Can you work these out from the model? Positions are in its coordinate system, mm. Give positions to 0.01 mm unless a question says otherwise; leave off trailing zeros. Order: outer loops, then holes, each group sorted by start corner. A loop starts at its lowest first (then second) coordinate and runs counter-clockwise, first axis right, second up. Notation, with made-up numbers: M 83,89.5 L 140,89.5 A22 ccw 140,107.5 Z; hole C -29.75,-4.75 d8. An arc over 180 degrees is marked long. One line per question, with ' | ' between items. Start each with the question number.
1) If we section it at D-D, the plane x = 46.5: Please give me the cut outline in (y, z), plus the area to 3 significant figures.
2) If we section it at A-A, the plane x = 34: Please give me the cut outline in (y, z).
3) If we section it at C-C, the plane y = 0.75: State how many separate pieces and enclosed holes the cut face has, plus the area to 3 significant figures.
4) If we section it at B-B, the plane x = 17: Please give me the cut outline in (y, z), plus the area to 3 significant figures.
5) Please list where these lines run through material, in increasing order: line 1 along Z through (x, y) = (23, 0.25); line 2 along Z through (x, y) = (26.5, 2.05); line 3 along X through (y, z) = (1.9, 38.5). Write a range as [from, to].
6) I'm going to push flat-ended pins straight in: pin 1 Ø1.5 at (x, y) = (30, 2) entering from -Z; pin 2 Ø1 at (y, z) = (2, -22) entering from +X; pin 3 Ø1.5 at (x, y) = (32.5, 1) entering from +Z. Where does each tip first touch, or does it pass through?
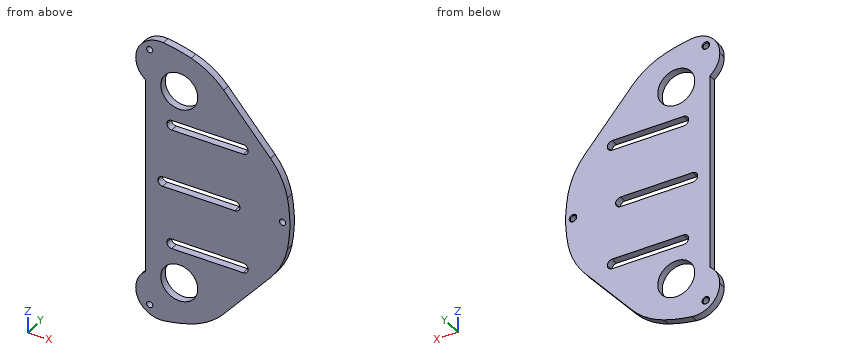
```python
from build123d import *

# Parameters (mm, degrees)
EXTRUDE_1_DEPTH              = 3
FILLET_1_R                   = 10
SKETCH_2_W                   = 33
SKETCH_2_H                   = 4
SKETCH_2_W_2                 = 33.308993126
CUT_EXTRUDE_1_DEPTH          = 83.523019213
SKETCH_3_W                   = 8
SKETCH_3_H                   = 80
CUT_EXTRUDE_2_DEPTH          = 83.523019213
FILLET_2_R                   = 10
FILLET_3_R                   = 2
CUT_EXTRUDE_3_DEPTH          = 83.523019213
FILLET_4_R                   = 30
SKETCH_5_R                   = 7.5
CUT_EXTRUDE_4_DEPTH          = 83.523019213
HOLE_WIZARD_M3_1_D           = 2.5
HOLE_WIZARD_M3_1_DEPTH       = 3
HOLE_WIZARD_M3_1_CSINK_D     = 3.05
HOLE_WIZARD_M3_1_CSINK_ANGLE = 90
HOLE_WIZARD_M3_1_TIP         = 0.751075774


# Some blends are built 0.0001 mm under size
with BuildPart() as part:
    # 草图1 → 凸台-拉伸1 (new body)
    with BuildSketch(Plane(origin=(0, 0, 0), x_dir=(1, 0, 0), z_dir=(0, 1, 0))):
        with BuildLine():
            Line((-4, 58.36308765), (-4, -58.36308765))
            ThreePointArc((-4, -58.36308765), (58.5, 0), (-4, 58.36308765))
        make_face()
    extrude(amount=EXTRUDE_1_DEPTH)

    # 圆角1
    fillet_1_edges = [part.edges().sort_by_distance(p)[0] for p in [
        (-4, 1.5, 58.36308765),
        (-4, 1.5, -58.36308765),
    ]]
    fillet(fillet_1_edges, radius=FILLET_1_R)

    # 草图2 → 切除-拉伸1 (cut, through all)
    with BuildSketch(Plane.XZ):
        with Locations((25.103538951, 24.75)):
            Rectangle(SKETCH_2_W, SKETCH_2_H)
        with Locations((25.103538951, -24.75)):
            Rectangle(SKETCH_2_W, SKETCH_2_H)
        with Locations((21.59426648, 0)):
            Rectangle(SKETCH_2_W_2, SKETCH_2_H)
    extrude(amount=-CUT_EXTRUDE_1_DEPTH, mode=Mode.SUBTRACT)

    # 草图3 → 切除-拉伸2 (cut, through all)
    with BuildSketch(Plane.XZ):
        with Locations((-4, 0)):
            Rectangle(SKETCH_3_W, SKETCH_3_H)
    extrude(amount=-CUT_EXTRUDE_2_DEPTH, mode=Mode.SUBTRACT)

    # 圆角2
    # the kernel refuses this fillet: 10 mm, written as the material it takes off along each edge
    with BuildSketch(Plane(origin=(-4, 23, 40), x_dir=(0, 0, 1), z_dir=(0, -1, 0)), Plane(origin=(-4, -20, -40), x_dir=(0, 0, -1), z_dir=(0, 1, 0))) as fillet_2_piece_1:
        with BuildLine():
            CenterArc((8, -10), FILLET_2_R, 90, 53.130102354)
            Line((0, -4), (-0.16, -3.88))
            ThreePointArc((-0.16, -3.88), (-0.2, -2), (-0.2, 0))
            Line((-0.2, 0), (0, 0.2))
            Line((0, 0.2), (8, 0.2))
            Line((8, 0.2), (8, 0))
        make_face()
    extrude(amount=43, mode=Mode.SUBTRACT)

    # 圆角3
    fillet_3_edges = [part.edges().sort_by_distance(p)[0] for p in [
        (8.603538951, 1.5, -26.75),
        (8.603538951, 1.5, -22.75),
        (41.603538951, 1.5, -26.75),
        (41.603538951, 1.5, -22.75),
        (4.939769917, 1.5, 2),
        (38.248763043, 1.5, 2),
        (38.248763043, 1.5, -2),
        (4.939769917, 1.5, -2),
        (41.603538951, 1.5, 22.75),
        (41.603538951, 1.5, 26.75),
        (8.603538951, 1.5, 22.75),
        (8.603538951, 1.5, 26.75),
    ]]
    fillet(fillet_3_edges, radius=FILLET_3_R - 0.0001)  # a hair under: the kernel refuses the full size

    # 草图4 → 切除-拉伸3 (cut, through all)
    with BuildSketch(Plane(origin=(0, 3, 0), x_dir=(1, 0, 0), z_dir=(0, 1, 0))):
        with BuildLine():
            Line((55.026651821, -19.857431591), (27.299740921, -51.73948343))
            ThreePointArc((27.299740921, -51.73948343), (44.142100571, -38.389125506), (55.026651821, -19.857431591))
        make_face()
        with BuildLine():
            Line((55.026651821, 19.857431591), (27.299740921, 51.73948343))
            ThreePointArc((27.299740921, 51.73948343), (44.142100571, 38.389125506), (55.026651821, 19.857431591))
        make_face()
    extrude(amount=-CUT_EXTRUDE_3_DEPTH, mode=Mode.SUBTRACT)

    # 圆角4
    fillet_4_edges = [part.edges().sort_by_distance(p)[0] for p in [
        (55.026651821, 1.5, 19.857431591),
        (27.299740921, 1.5, 51.73948343),
        (27.299740921, 1.5, -51.73948343),
        (55.026651821, 1.5, -19.857431591),
    ]]
    fillet(fillet_4_edges, radius=FILLET_4_R)

    # 草图5 → 切除-拉伸4 (cut, through all)
    with BuildSketch(Plane(origin=(0, 3, 0), x_dir=(1, 0, 0), z_dir=(0, 1, 0))):
        with Locations(Location((13.650269614, 40, 0), (0, 0, 270))):
            Circle(SKETCH_5_R)
        with Locations(Location((13.650269614, -40, 0), (0, 0, 270))):
            Circle(SKETCH_5_R)
    extrude(amount=-CUT_EXTRUDE_4_DEPTH, mode=Mode.SUBTRACT)

    # M3 螺纹孔1
    with Locations(Plane(origin=(0, 3, 0), x_dir=(1, 0, 0), z_dir=(0, 1, 0))):
        with Locations((1.668639438, 53.213363577), (1.668639438, -53.213363577), (0.79229906, -68.463573452), (55.526064592, 0.086594156)):
            CounterSinkHole(HOLE_WIZARD_M3_1_D / 2, HOLE_WIZARD_M3_1_CSINK_D / 2, depth=HOLE_WIZARD_M3_1_DEPTH, counter_sink_angle=HOLE_WIZARD_M3_1_CSINK_ANGLE)
            with Locations((0, 0, -(HOLE_WIZARD_M3_1_DEPTH + HOLE_WIZARD_M3_1_TIP / 2))):  # 118° drill point
                Cone(0, HOLE_WIZARD_M3_1_D / 2, HOLE_WIZARD_M3_1_TIP, mode=Mode.SUBTRACT)


solid = part.part
```
Results found:
1) outline: M 0,-29.66 L 3,-29.66 L 3,29.66 L 0,29.66 Z | area: 178 mm²
2) outline: M 0,-44.04 L 3,-44.04 L 3,-26.75 L 0,-26.75 Z; M 0,-22.75 L 3,-22.75 L 3,-2 L 0,-2 Z; M 0,2 L 3,2 L 3,22.75 L 0,22.75 Z; M 0,26.75 L 3,26.75 L 3,44.04 L 0,44.04 Z
3) separate pieces: 1 | enclosed holes: 8 | area: 4,460 mm²
4) outline: M 0,-55.98 L 3,-55.98 L 3,-46.71 L 0,-46.71 Z; M 0,-33.29 L 3,-33.29 L 3,-26.75 L 0,-26.75 Z; M 0,-22.75 L 3,-22.75 L 3,-2 L 0,-2 Z; M 0,2 L 3,2 L 3,22.75 L 0,22.75 Z; M 0,26.75 L 3,26.75 L 3,33.29 L 0,33.29 Z; M 0,46.71 L 3,46.71 L 3,55.98 L 0,55.98 Z | area: 219 mm²
5) line 1: z = [-53.58, -26.75], [-22.75, -2], [2, 22.75], [26.75, 53.58] | line 2: z = [-51.42, -26.75], [-22.75, -2], [2, 22.75], [26.75, 51.42] | line 3: x = [0, 6.3], [21, 38.81]
6) pin 1: stops at z = -49.19 | pin 2: stops at x = 53.2 | pin 3: stops at z = 46.62
